CAD build for the part. Positions are in the model's coordinates, mm. Face numbers are marked on the shaded views. A direction names the side the tool comes from. Coordinates: 2 decimals unless noted, no trailing zeros. Loops run counter-clockwise (first coordinate to the right, second up) from the corner with the lowest first, then second, coordinate; pieces in that order, holes last. Notation, with made-up numbers: (2, -27) -> (58, -27) arc R16 cw to (58, 0) -> close; hole circle Ø11 at (-8.75, 18.25). An arc over 180 degrees is marked (long way). Answer as a JSON object with one key per item and string values. Group by question number.
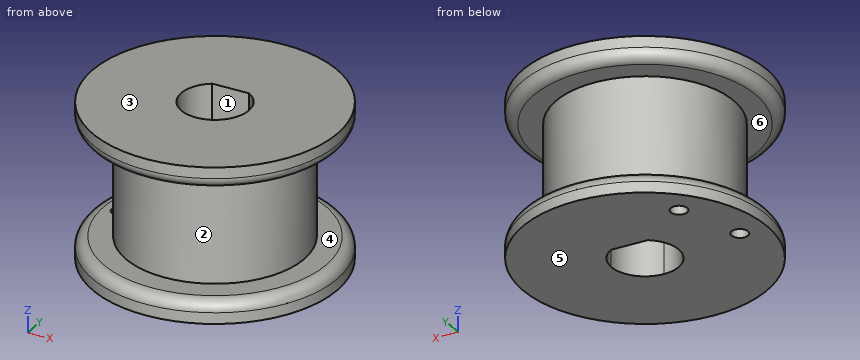
from build123d import *

# Parameters (mm, degrees)
F0_R     = 8.05
F1_DEPTH = 14
F0_R_2   = 11.05
F2_DEPTH = 14
F3_DEPTH = 12
F4_DEPTH = 2
F5_R     = 1
F6_D     = 1.5
F6_DEPTH = 2
F6_TIP   = 0.4506454643
F7_D     = 1.5
F7_DEPTH = 2
F7_TIP   = 0.4506454643


with BuildPart() as f1:
    # F0 (on Top) → F1 (new body)
    with BuildSketch(Plane.XY):
        Circle(F0_R)
        with BuildLine():
            ThreePointArc((1.6733200531, 2.55), (2.6838522837, 1.4489433802), (3.05, 0))
            ThreePointArc((3.05, 0), (2.1566756826, -2.1566756826), (0, -3.05))
            ThreePointArc((0, -3.05), (-2.9223278392, -0.8732124598), (-1.6733200531, 2.55))
            ThreePointArc((-1.6733200531, 2.55), (0, 3.05), (1.6733200531, 2.55))
        make_face(mode=Mode.SUBTRACT)
        with BuildLine():
            Line((0, 2.55), (1.6733200531, 2.55))
            ThreePointArc((1.6733200531, 2.55), (0, 3.05), (-1.6733200531, 2.55))
            Line((-1.6733200531, 2.55), (0, 2.55))
        make_face()
    extrude(amount=F1_DEPTH)

    # F0 (on Top) → F2 (join)
    with BuildSketch(Plane.XY):
        Circle(F0_R_2)
        Circle(F0_R, mode=Mode.SUBTRACT)
    extrude(amount=F2_DEPTH)

    # F0 (on Top) → F3 (cut)
    with BuildSketch(Plane.XY):
        Circle(F0_R_2)
        Circle(F0_R, mode=Mode.SUBTRACT)
    extrude(amount=F3_DEPTH, mode=Mode.SUBTRACT)

    # F0 (on Top) → F4 (join)
    with BuildSketch(Plane.XY):
        Circle(F0_R_2)
        Circle(F0_R, mode=Mode.SUBTRACT)
    extrude(amount=F4_DEPTH)

    # F5
    f5_edges = [f1.edges().sort_by_distance(p)[0] for p in [
        (-11.05, 0, 12),
        (-11.05, 0, 2),
    ]]
    fillet(f5_edges, radius=F5_R)

    # F6
    with Locations(Plane(origin=(0, 0, 0), x_dir=(1, 0, 0), z_dir=(0, 0, -1))):
        with Locations((-8.5659669712, 0)):
            Hole(F6_D / 2, depth=F6_DEPTH)
            with Locations((0, 0, -(F6_DEPTH + F6_TIP / 2))):  # 118° drill point
                Cone(0, F6_D / 2, F6_TIP, mode=Mode.SUBTRACT)

    # F7
    with Locations(Plane(origin=(0, 0, 0), x_dir=(1, 0, 0), z_dir=(0, 0, -1))):
        with Locations((-6.2731071375, -5.7528195903)):
            Hole(F7_D / 2, depth=F7_DEPTH)
            with Locations((0, 0, -(F7_DEPTH + F7_TIP / 2))):  # 118° drill point
                Cone(0, F7_D / 2, F7_TIP, mode=Mode.SUBTRACT)


solid = f1.part
Item 1: Drill centre lines: L1, parallel to Z at x = 2.25, y = 8.5; L2, parallel to Y at x = 0, z = 5.5; L3, parallel to X at y = 0.25, z = 1. Where is each one in solid material? Low to high.
Item 2: Band-saw the part on A-A, the plane z = 2.5. List the corners of the cut face in (x, y), and give its area (3 significant figures).
Item 3: Pull direction Z, two halves, no side cores. Call the marked faces 1, 2, 3 and 4: +Z half, -Z half, draft (parallel to the pull), parting line (faces both ways), or undercut.
Item 4: 3-axis set-ups, long thin cutter, end or side, ignore diameter. For the marked faces 5 and 6: which of +Z, -Z, +X, -X, +Y, -Y reach the whole face in a straight line?
Item 5: Flat gauge pins, fed straight in: P1, Ø3, axis at x = 5, z = 5.5, coming from the -Y side; P2, Ø8, axis at x = -7, z = 2.5, coming from the -Y side; P3, Ø1.5, axis at x = -4, z = 5.5, coming from the +Y side; P4, Ø2.5, axis at x = -8.57, y = 0, coming from the -Z side. Where does each tip first touch, or does it go through?
Reply:
{
 "1": {"L1": "0 to 2, 12 to 14", "L2": "-8.05 to -3.05, 2.55 to 8.05", "L3": "-11.05 to -9.27, -7.86 to -3.04, 3.04 to 11.05"},
 "2": {"outline": "circle Ø16.1 at (0, 0); hole (-1.67, 2.55) arc R3.05 ccw (long way) to (1.67, 2.55) -> close", "area": "175 mm²"},
 "3": {"face 1": "draft", "face 2": "undercut", "face 3": "+Z half", "face 4": "undercut"},
 "4": {"face 5": "-Z, +X, -X, +Y, -Y", "face 6": "none"},
 "5": {"P1": "y = -7.25", "P2": "y = -10.56", "P3": "y = 7.36", "P4": "z = 0"}
}
